from build123d import *

# Parameters (mm, degrees)
SKIZZE1_R                       = 95
SKIZZE1_R_2                     = 1.6
AUFSATZ_LINEAR_AUSTRAGEN1_DEPTH = 3
SKIZZE2_W                       = 70
SKIZZE2_H                       = 4
SCHNITT_LINEAR_AUSTRAGEN2_DEPTH = 3
VERRUNDUNG1_R                   = 1


with BuildPart() as part:
    # Skizze1 → Aufsatz-Linear austragen1 (new body)
    with BuildSketch(Plane(origin=(0, 0, 0), x_dir=(1, 0, 0), z_dir=(0, 1, 0))):
        with Locations(Location((0, 0, 0), (0, 0, 270))):
            Circle(SKIZZE1_R)
        with Locations(Location((-52, 68, 0), (0, 0, 270))):
            Circle(SKIZZE1_R_2, mode=Mode.SUBTRACT)
        with Locations(Location((52, 68, 0), (0, 0, 270))):
            Circle(SKIZZE1_R_2, mode=Mode.SUBTRACT)
        with Locations(Location((-52, -68, 0), (0, 0, 270))):
            Circle(SKIZZE1_R_2, mode=Mode.SUBTRACT)
        with Locations(Location((52, -68, 0), (0, 0, 270))):
            Circle(SKIZZE1_R_2, mode=Mode.SUBTRACT)
        with BuildLine():
            Line((-44, 65), (-44, -65))
            ThreePointArc((-44, -65), (-43.121320344, -67.121320344), (-41, -68))
            Line((-41, -68), (41, -68))
            ThreePointArc((41, -68), (43.121320344, -67.121320344), (44, -65))
            Line((44, -65), (44, 65))
            ThreePointArc((44, 65), (43.121320344, 67.121320344), (41, 68))
            Line((41, 68), (-41, 68))
            ThreePointArc((-41, 68), (-43.121320344, 67.121320344), (-44, 65))
        make_face(mode=Mode.SUBTRACT)
    extrude(amount=AUFSATZ_LINEAR_AUSTRAGEN1_DEPTH)

    # Skizze2 → Schnitt-Linear austragen2 (cut)
    with BuildSketch(Plane(origin=(0, 0, 0), x_dir=(1, 0, 0), z_dir=(0, 1, 0))):
        with Locations((0, -68)):
            Rectangle(SKIZZE2_W, SKIZZE2_H)
        with Locations((0, 68)):
            Rectangle(SKIZZE2_W, SKIZZE2_H)
    extrude(amount=SCHNITT_LINEAR_AUSTRAGEN2_DEPTH, mode=Mode.SUBTRACT)

    # Verrundung1
    verrundung1_edges = [part.edges().sort_by_distance(p)[0] for p in [
        (-35, 1.5, 70),
        (35, 1.5, 70),
        (35, 1.5, -70),
        (-35, 1.5, -70),
    ]]
    fillet(verrundung1_edges, radius=VERRUNDUNG1_R)
    verrundung1_2_edges = [part.edges().sort_by_distance(p)[0] for p in [
        (-35, 1.5, 68),
        (35, 1.5, 68),
        (35, 1.5, -68),
        (-35, 1.5, -68),
    ]]
    fillet(verrundung1_2_edges, radius=VERRUNDUNG1_R - 0.0001)  # a hair under: the kernel refuses the full size


solid = part.part
Part model, mm, in its own coordinate system. Round coordinates to 2 decimals unless told otherwise and drop trailing zeros. Write each loop counter-clockwise with the first axis right and the second up, starting at its lowest first coordinate (ties: lowest second). Pieces come first, ordered by that corner, then holes. Notation, with made-up numbers: M 25,25 L 73,25 A20 cw 73,34 Z; hole C 2.5,54.5 d2. An arc over 180 degrees is marked long. Return JSON: item names as keys, results as strings. Group by question number.
(1) Drill centre lines: probe 1 along X at (y, z) = (2.1, 30.5); probe 2 along Z at (x, y) = (34.5, 2.85); probe 3 along X at (y, z) = (2.7, -7.5). Where is each one in solid material? Low to high.
(2) Saw through at A-A on z = 0. Write the cut outline in (x, y), then the cut area to 3 significant figures.
(3) Saw through at C-C on y = 2.15. Count the separate pieces of the cut face and the enclosed holes in it, then the cut area to 3 significant figures.
(4) Saw through at D-D on x = -56.5. Write the cut outline in (y, z).
(5) Saw through at B-B on x = 7.5. Write the cut outline in (y, z).
(6) Pin check, flat tips, straight feed: pin 1 Ø1.5 at (x, y) = (-48, 2) entering from -Z; pin 2 Ø1.5 at (x, y) = (-39, 1.5) entering from -Z; pin 3 Ø1.5 at (x, y) = (-39, 1) entering from +Z. Stop position of each tip, or through.
Returned:
{
 "1": {"probe 1": "-89.97 to -44, 44 to 89.97", "probe 2": "-88.51 to -69.87, 69.87 to 88.51", "probe 3": "-94.7 to -44, 44 to 94.7"},
 "2": {"outline": "M -95,0 L -44,0 L -44,3 L -95,3 Z; M 44,0 L 95,0 L 95,3 L 44,3 Z", "area": "306 mm²"},
 "3": {"separate pieces": "1", "enclosed holes": "5", "area": "16,100 mm²"},
 "4": {"outline": "M 0,-76.37 L 3,-76.37 L 3,76.37 L 0,76.37 Z"},
 "5": {"outline": "M 0,-94.7 L 3,-94.7 L 3,-70 L 0,-70 Z; M 0,70 L 3,70 L 3,94.7 L 0,94.7 Z"},
 "6": {"pin 1": "z = -82.42", "pin 2": "z = -86.96", "pin 3": "z = 86.96"}
}
